from build123d import *

# Parameters (mm, degrees)
SKETCH_1_R          = 8
EXTRUDE_1_DEPTH     = 16
SKETCH_2_W          = 2
SKETCH_2_H          = 16
CUT_EXTRUDE_1_DEPTH = 16
SKETCH_3_R          = 2
CUT_EXTRUDE_2_DEPTH = 39
SKETCH_4_R          = 1.5
CUT_EXTRUDE_3_DEPTH = 39


with BuildPart() as part:
    # 草图1 → 凸台-拉伸1 (new body)
    with BuildSketch(Plane.XY):
        Polygon((-24.921659643, 3.123294018), (19.078340357, 3.123294018), (19.078340357, 11.123294018), (9.578340357, 11.123294018), (9.578340357, 47.123294018), (-15.421659643, 47.123294018), (-15.421659643, 11.123294018), (-24.921659643, 11.123294018), align=None)
        with Locations((-2.921659643, 30.123294018)):
            Circle(SKETCH_1_R, mode=Mode.SUBTRACT)
    extrude(amount=EXTRUDE_1_DEPTH)

    # 草图2 → 切除-拉伸1 (cut)
    with BuildSketch(Plane(origin=(0, 47.123294018, 0), x_dir=(1, 0, 0), z_dir=(0, 1, 0))):
        with Locations((-2.921659643, -8)):
            Rectangle(SKETCH_2_W, SKETCH_2_H)
    extrude(amount=-CUT_EXTRUDE_1_DEPTH, mode=Mode.SUBTRACT)

    # 草图3 → 切除-拉伸2 (cut)
    with BuildSketch(Plane(origin=(9.578340357, 0, 0), x_dir=(0, 0, -1), z_dir=(1, 0, 0))):
        with Locations((-8, 42.123294018)):
            Circle(SKETCH_3_R)
    extrude(amount=-CUT_EXTRUDE_2_DEPTH, mode=Mode.SUBTRACT)

    # 草图4 → 切除-拉伸3 (cut)
    with BuildSketch(Plane.XZ.offset(-3.123294018)):
        with Locations((-21.921659643, 8)):
            Circle(SKETCH_4_R)
        with Locations((16.078340357, 8)):
            Circle(SKETCH_4_R)
    extrude(amount=-CUT_EXTRUDE_3_DEPTH, mode=Mode.SUBTRACT)


solid = part.part
Could you check a few things on this model? Use its own coordinates, in mm. A direction names the side the tool comes from. Give positions to 0.01 mm unless a question says otherwise; leave off trailing zeros. Order: outer loops, then holes, each group sorted by start corner. A loop starts at its lowest first (then second) coordinate and runs counter-clockwise, first axis right, second up. Notation, with made-up numbers: (-8.75, 82) -> (19.25, 82) arc R14 ccw to (19.25, 96) -> close; hole circle Ø3 at (-17.75, -1.75). An arc over 180 degrees is marked (long way). Answer in a Markdown table with one row per item. Add a question column.
Item 1: For faces 4 (the cylindrical face through (-9.6, 44.1, 8.3)), 5 (the flat face through (-20, 11.123, 8)), 6 (the flat face through (9.578, 29, 8)), 7 (the flat face through (-3.922, 45, 8)), 8 (the flat face through (19.078, 7, 8)), which set-ups out of +Z, -Z, +X, -X, +Y, -Y let a thin tool reach every point of the face, with its end or its side?
Item 2: Imagine slicing it at D-D (z = 3). List the corners of the cut face in (x, y) for me.
Item 3: Imagine slicing it at C-C (x = -10). List the corners of the cut face in (y, z) for me, and give its area (3 significant figures).
Item 4: Imagine slicing it at B-B (z = 8). List the corners of the cut face in (x, y) for me.
Item 5: Please list where these lines run through material, in increasing order: probe 1 along X at (y, z) = (45.5, 3.5); probe 2 along X at (y, z) = (14, 15.75); probe 3 along Y at (x, z) = (-19, 3.25).
Item 6: Imagine slicing it at A-A (y = 25). List the corners of the cut face in (x, z) for me, and give its area (3 significant figures).
Item 7: We'd pull the mould along Y, two halves only. Please class faces 1 (the cylindrical face through (-20.536, 7.067, 7.425)), 2 (the flat face through (-10, 47.123, 8)), 3 (the cylindrical face through (-3.26, 22.13, 7.89)): pulls with the +Y half, pulls with the -Y half, needs draft (parallel to the pull), parting line crosses it, or undercut.
Item 8: I'm going to push flat-ended pins straight in: P1, Ø5, axis at y = 36.5, z = 8.5, coming from the +X side; P2, Ø1, axis at y = 25, z = 3.5, coming from the -X side; P3, Ø5, axis at x = 16.08, z = 8, coming from the +Y side. Where does each tip first touch, or does it pass through?
Result:
| question | item | result |
|---|---|---|
| 1 | face 4 | +X, -X |
| 1 | face 5 | +Z, -Z, -X, +Y |
| 1 | face 6 | +Z, -Z, +X, +Y |
| 1 | face 7 | +Z, -Z, +Y |
| 1 | face 8 | +Z, -Z, +X, +Y, -Y |
| 2 | outline | (-24.92, 3.12) -> (19.08, 3.12) -> (19.08, 11.12) -> (9.58, 11.12) -> (9.58, 47.12) -> (-1.92, 47.12) -> (-1.92, 38.06) arc R8 cw (long way) to (-3.92, 38.06) -> (-3.92, 47.12) -> (-15.42, 47.12) -> (-15.42, 11.12) -> (-24.92, 11.12) -> close |
| 3 | outline | (3.12, 0) -> (26.4, 0) -> (26.4, 16) -> (3.12, 16) -> close; (33.85, 0) -> (47.12, 0) -> (47.12, 16) -> (33.85, 16) -> close; hole circle Ø4 at (42.12, 8) |
| 3 | area | 572 mm2 |
| 4 | outline | (-24.92, 3.12) -> (-23.42, 3.12) -> (-23.42, 11.12) -> (-24.92, 11.12) -> close; (-20.42, 3.12) -> (14.58, 3.12) -> (14.58, 11.12) -> (9.58, 11.12) -> (9.58, 40.12) -> (-1.92, 40.12) -> (-1.92, 38.06) arc R8 cw (long way) to (-3.92, 38.06) -> (-3.92, 40.12) -> (-15.42, 40.12) -> (-15.42, 11.12) -> (-20.42, 11.12) -> close; (-15.42, 44.12) -> (-3.92, 44.12) -> (-3.92, 47.12) -> (-15.42, 47.12) -> close; (-1.92, 44.12) -> (9.58, 44.12) -> (9.58, 47.12) -> (-1.92, 47.12) -> close; (17.58, 3.12) -> (19.08, 3.12) -> (19.08, 11.12) -> (17.58, 11.12) -> close |
| 5 | probe 1 | -15.42 to -3.92, -1.92 to 9.58 |
| 5 | probe 2 | -15.42 to 9.58 |
| 5 | probe 3 | 3.12 to 11.12 |
| 6 | outline | (-15.42, 0) -> (-9.07, 0) -> (-9.07, 16) -> (-15.42, 16) -> close; (3.22, 0) -> (9.58, 0) -> (9.58, 16) -> (3.22, 16) -> close |
| 6 | area | 203 mm2 |
| 7 | face 1 | needs draft |
| 7 | face 2 | pulls with the +Y half |
| 7 | face 3 | undercut |
| 8 | P1 | x = 9.58 |
| 8 | P2 | x = -15.42 |
| 8 | P3 | y = 11.12 |
